Part model, mm, in its own coordinate system. Face numbers are marked on the shaded views. Round coordinates to 2 decimals unless told otherwise and drop trailing zeros. Order: outer loops, then holes, each group sorted by start corner. A loop starts at its lowest first (then second) coordinate and runs counter-clockwise, first axis right, second up. Notation, with made-up numbers: (-23.75, -13.75) - (11.25, -13.75) arc R20 ccw to (11.25, 0.25) - close; hole circle Ø10 at (-4, -26). An arc over 180 degrees is marked (long way). Return JSON: item names as keys, results as strings. Group by question number.
Item 1: Two-plate mould, pull along Y, no slides. Class the marked faces 1, 2 and 3: released by +Y, released by -Y, zero draft, split by the parting line, or undercut.
Item 2: Saw through at B-B on z = -19.05. List the corners of the cut face in (x, y).
Item 3: Saw through at D-D on x = 0. State how many separate pieces and enclosed holes the cut face has, and give its area (3 significant figures).
Item 4: Saw through at C-C on y = 8. List the corners of the cut face in (x, z) (3 decimals), and give its area (3 significant figures).
Item 5: Saw through at A-A on x = 19.05. List the corners of the cut face in (y, z).
Item 6: Probe probe 1 along Y at (x, z) = (18, 2.5); probe 2 along X at (y, z) = (99, 0) (3 decimals); probe 3 along X at (y, z) = (96.5, 19.05). List the from-to ranges inside material, lowest first.
Item 7: Drop flat-ended pins along their axis: pin 1 (8 mm diameter, centred on y = 56, z = 9.5, fed in from -X); pin 2 (1.4 mm diameter, centred on x = 19.05, z = 0, fed in from +Y); pin 3 (6 mm diameter, centred on x = -14.5, z = -3, fed in from -Y); pin 4 (3 mm diameter, centred on x = 1, y = 64.5, fed in from +Z). Give the stop position or say it passes through.
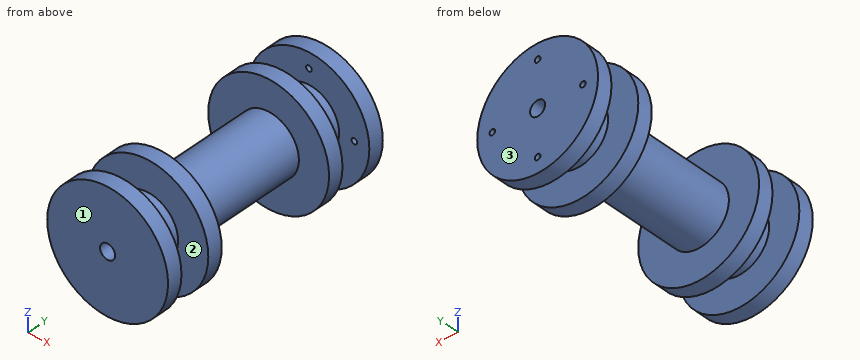
```python
from build123d import *

# Parameters (mm, degrees)
SKETCH1_R           = 25.4
BOSS_EXTRUDE1_DEPTH = 101.6
SKETCH2_W           = 12.7
SKETCH2_H           = 12.7
SKETCH2_H_2         = 50.8
CUT_EXTRUDE1_REACH  = 109.763
SKETCH3_R           = 3.175
CUT_EXTRUDE2_REACH  = 109.763
SKETCH4_R           = 1.18745


with BuildPart() as part:
    # Sketch1 → Boss-Extrude1 (new body)
    with BuildSketch(Plane(origin=(0, 0, 0), x_dir=(1, 0, 0), z_dir=(0, 1, 0))):
        with Locations(Location((0, 0, 0), (0, 0, 270))):
            Circle(SKETCH1_R)
    extrude(amount=BOSS_EXTRUDE1_DEPTH)

    # Sketch2 → Cut-Revolve1 (revolve, cut)
    with BuildSketch(Plane(origin=(0, 0, 0), x_dir=(0, 0, -1), z_dir=(1, 0, 0)), mode=Mode.PRIVATE) as cut_revolve1_sk:
        with Locations((19.05, 88.9)):
            Rectangle(SKETCH2_W, SKETCH2_H)
        with Locations((19.05, 12.7)):
            Rectangle(SKETCH2_W, SKETCH2_H)
        with Locations((19.05, 50.8)):
            Rectangle(SKETCH2_W, SKETCH2_H_2)
    revolve(cut_revolve1_sk.sketch.rotate(Axis((0, 101.6, 0), (0, -1, 0)), 180), axis=Axis((0, 101.6, 0), (0, -1, 0)), mode=Mode.SUBTRACT)

    # Sketch3 → Cut-Extrude1 (cut, up to next)
    with BuildSketch(Plane(origin=(0, 101.6, 0), x_dir=(1, 0, 0), z_dir=(0, 1, 0)), mode=Mode.PRIVATE) as cut_extrude1_sk1:
        with Locations(Location((0, 0, 0), (0, 0, 270))):
            Circle(SKETCH3_R)
    cut_extrude1_tool1 = extrude(cut_extrude1_sk1.sketch, amount=-CUT_EXTRUDE1_REACH, mode=Mode.PRIVATE) & part.part
    add(cut_extrude1_tool1.solids().sort_by_distance((0, 101.6, 0))[0], mode=Mode.SUBTRACT)

    # Sketch4 → Cut-Extrude2 (cut, up to next)
    with BuildSketch(Plane(origin=(0, 101.6, 0), x_dir=(1, 0, 0), z_dir=(0, 1, 0)), mode=Mode.PRIVATE) as cut_extrude2_sk1:
        with Locations(Location((-19.05, 0, 0), (0, 0, 270))):
            Circle(SKETCH4_R)
    cut_extrude2_tool1 = extrude(cut_extrude2_sk1.sketch, amount=-CUT_EXTRUDE2_REACH, mode=Mode.PRIVATE) & part.part
    # Sketch4 → Cut-Extrude2 (cut, up to next)
    with BuildSketch(Plane(origin=(0, 101.6, 0), x_dir=(1, 0, 0), z_dir=(0, 1, 0)), mode=Mode.PRIVATE) as cut_extrude2_sk2:
        with Locations(Location((0, 19.05, 0), (0, 0, 270))):
            Circle(SKETCH4_R)
    cut_extrude2_tool2 = extrude(cut_extrude2_sk2.sketch, amount=-CUT_EXTRUDE2_REACH, mode=Mode.PRIVATE) & part.part
    # Sketch4 → Cut-Extrude2 (cut, up to next)
    with BuildSketch(Plane(origin=(0, 101.6, 0), x_dir=(1, 0, 0), z_dir=(0, 1, 0)), mode=Mode.PRIVATE) as cut_extrude2_sk3:
        with Locations(Location((19.05, 0, 0), (0, 0, 270))):
            Circle(SKETCH4_R)
    cut_extrude2_tool3 = extrude(cut_extrude2_sk3.sketch, amount=-CUT_EXTRUDE2_REACH, mode=Mode.PRIVATE) & part.part
    # Sketch4 → Cut-Extrude2 (cut, up to next)
    with BuildSketch(Plane(origin=(0, 101.6, 0), x_dir=(1, 0, 0), z_dir=(0, 1, 0)), mode=Mode.PRIVATE) as cut_extrude2_sk4:
        with Locations(Location((0, -19.05, 0), (0, 0, 270))):
            Circle(SKETCH4_R)
    cut_extrude2_tool4 = extrude(cut_extrude2_sk4.sketch, amount=-CUT_EXTRUDE2_REACH, mode=Mode.PRIVATE) & part.part
    add(cut_extrude2_tool1.solids().sort_by_distance((-19.05, 101.6, 0))[0], mode=Mode.SUBTRACT)
    add(cut_extrude2_tool2.solids().sort_by_distance((0, 101.6, -19.05))[0], mode=Mode.SUBTRACT)
    add(cut_extrude2_tool3.solids().sort_by_distance((19.05, 101.6, 0))[0], mode=Mode.SUBTRACT)
    add(cut_extrude2_tool4.solids().sort_by_distance((0, 101.6, 19.05))[0], mode=Mode.SUBTRACT)


solid = part.part
```
Filled in:
{
 "1": {"face 1": "released by -Y", "face 2": "undercut", "face 3": "released by +Y"},
 "2": {"outline": "(-16.8, 0) - (16.8, 0) - (16.8, 6.35) - (-16.8, 6.35) - close; (-16.8, 19.05) - (16.8, 19.05) - (16.8, 25.4) - (-16.8, 25.4) - close; (-16.8, 76.2) - (16.8, 76.2) - (16.8, 82.55) - (-16.8, 82.55) - close; (-16.8, 95.25) - (-1.19, 95.25) - (-1.19, 101.6) - (-16.8, 101.6) - close; (1.19, 95.25) - (16.8, 95.25) - (16.8, 101.6) - (1.19, 101.6) - close"},
 "3": {"separate pieces": "4", "enclosed holes": "0", "area": "2,550 mm^2"},
 "4": {"outline": "circle Ø25.4 at (0, 0); hole circle Ø6.35 at (0, 0)", "area": "475 mm^2"},
 "5": {"outline": "(0, -16.8) - (6.35, -16.8) - (6.35, 16.8) - (0, 16.8) - close; (19.05, -16.8) - (25.4, -16.8) - (25.4, 16.8) - (19.05, 16.8) - close; (76.2, -16.8) - (82.55, -16.8) - (82.55, 16.8) - (76.2, 16.8) - close; (95.25, -16.8) - (101.6, -16.8) - (101.6, -1.19) - (95.25, -1.19) - close; (95.25, 1.19) - (101.6, 1.19) - (101.6, 16.8) - (95.25, 16.8) - close"},
 "6": {"probe 1": "y = 0 to 6.35, 19.05 to 25.4, 76.2 to 82.55, 95.25 to 101.6", "probe 2": "x = -25.4 to -20.237, -17.863 to -3.175, 3.175 to 17.863, 20.237 to 25.4", "probe 3": "x = -16.8 to -1.19, 1.19 to 16.8"},
 "7": {"pin 1": "stops at x = -11.45", "pin 2": "stops at y = 82.55", "pin 3": "stops at y = 0", "pin 4": "stops at z = 12.7"}
}
